```python
from build123d import *

# Parameters (mm, degrees)
F2_DEPTH = 200
F3_W     = 5
F3_H     = 20
F4_DEPTH = 5
F5_W     = 5
F5_H     = 20
F6_DEPTH = 5
F7_D     = 5


with BuildPart() as f2:
    # F1 (on Top) → F2 (new body)
    with BuildSketch(Plane.XY):
        Polygon((30, -55), (30, -15), (25, -15), (25, -50), (-25, -50), (-25, -15), (-30, -15), (-30, -55), align=None)
    extrude(amount=F2_DEPTH)

    # F3 (on face) → F4 (join)
    with BuildSketch(Plane.YZ.offset(30)):
        with Locations((-12.5, 150)):
            Rectangle(F3_W, F3_H)
        with Locations((-12.5, 40)):
            Rectangle(F3_W, F3_H)
    extrude(amount=-F4_DEPTH)

    # F5 (on face) → F6 (join)
    with BuildSketch(Plane(origin=(-30, 0, 0), x_dir=(0, -1, 0), z_dir=(-1, 0, 0))):
        with Locations((12.5, 150)):
            Rectangle(F5_W, F5_H)
        with Locations((12.5, 40)):
            Rectangle(F5_W, F5_H)
    extrude(amount=-F6_DEPTH)

    # F7 (through all)
    with Locations(Plane.YZ.offset(30)):
        with Locations((-25, 150), (-25, 40)):
            Hole(F7_D / 2)


solid = f2.part
```
Input: part model. Units: mm. Frame: model coordinates. A direction names the side the tool comes from. Coordinates: 2 decimals unless noted, no trailing zeros. Loops run counter-clockwise (first coordinate to the right, second up) from the corner with the lowest first, then second, coordinate; pieces in that order, holes last. Notation, with made-up numbers: M -37,-24.5 L 18,-24.5 A19 cw 18,10.5 Z; hole C -33,42 d10. An arc over 180 degrees is marked long. Use a Markdown table: item, result. Add a question column.
1) Pin query (flat end, axial travel): P1, Ø1.5, axis at x = 26.5, z = 14, coming from the +Y side; P2, Ø25, axis at x = 8.5, z = 141.5, coming from the +Y side; P3, Ø2, axis at x = 17.5, y = -50, coming from the -Z side; P4, Ø1.5, axis at x = -27, y = -12.5, coming from the -Z side. Return the tip coordinate at first contact, or that it passes through.
2) Section C-C, the plane y = -25. Return the cut outline in (x, z).
3) Line query: L1, parallel to Z at x = -28.45, y = -25; L2, parallel to X at y = -15, z = 141; L3, parallel to Y at x = -26.15, z = 150. Output: solid intervals per line, ascending. Write a range as from..to.
4) Section B-B, the plane z = 150. Return the cut outline in (x, y), plus the area to 3 significant figures.
5) Set-up query: faces 1 (the flat face through (-27, -15, 94)), 2 (the flat face through (-27, -15, 180)), 3 (the flat face through (0, -50, 99)), 4 (the cylindrical face through (-27.54, -24.46, 37.56)), 5 (the flat face through (28, -15, 15)). Return all of +Z, -Z, +X, -X, +Y, -Y with unobstructed straight access to the full face (end or side cutting, diameter ignored); none if empty.
6) Section D-D, the plane z = 122. Return the cut outline in (x, y), plus the area to 3 significant figures.
7) Section A-A, the plane y = -44. Return the cut outline in (x, z), plus the area to 3 significant figures.
8) Draft query along Y for faces 6 (the cylindrical face through (27.47, -24.67, 152.48)), 7 (the flat face through (28, -13, 140)), 8 (the flat face through (-27, -15, 15)). Return one class per face: +Y half, -Y half, draft (parallel to the pull), parting line (faces both ways), or undercut.
Answer below:
| question | item | result |
|---|---|---|
| 1 | P1 | y = -15 |
| 1 | P2 | y = -50 |
| 1 | P3 | z = 0 |
| 1 | P4 | z = 30 |
| 2 | outline | M -30,0 L -25,0 L -25,37.5 L -30,37.5 Z; M -30,42.5 L -25,42.5 L -25,147.5 L -30,147.5 Z; M -30,152.5 L -25,152.5 L -25,200 L -30,200 Z; M 25,0 L 30,0 L 30,37.5 L 25,37.5 Z; M 25,42.5 L 30,42.5 L 30,147.5 L 25,147.5 Z; M 25,152.5 L 30,152.5 L 30,200 L 25,200 Z |
| 3 | L1 | 0..37.5, 42.5..147.5, 152.5..200 |
| 3 | L2 | -30..-25, 25..30 |
| 3 | L3 | -55..-27.5, -22.5..-10 |
| 4 | outline | M -30,-55 L 30,-55 L 30,-27.5 L 25,-27.5 L 25,-50 L -25,-50 L -25,-27.5 L -30,-27.5 Z; M -30,-22.5 L -25,-22.5 L -25,-10 L -30,-10 Z; M 25,-22.5 L 30,-22.5 L 30,-10 L 25,-10 Z |
| 4 | area | 650 mm2 |
| 5 | face 1 | +X, -X, +Y |
| 5 | face 2 | +Z, +X, -X, +Y |
| 5 | face 3 | +Z, -Z, +Y |
| 5 | face 4 | +X, -X |
| 5 | face 5 | -Z, +X, -X, +Y |
| 6 | outline | M -30,-55 L 30,-55 L 30,-15 L 25,-15 L 25,-50 L -25,-50 L -25,-15 L -30,-15 Z |
| 6 | area | 650 mm2 |
| 7 | outline | M -30,0 L -25,0 L -25,200 L -30,200 Z; M 25,0 L 30,0 L 30,200 L 25,200 Z |
| 7 | area | 2,000 mm2 |
| 8 | face 6 | undercut |
| 8 | face 7 | draft |
| 8 | face 8 | +Y half |
